Input: dimensioned drawing with shaded views. Units: mm. Origin: part minimum x, y, z. Coordinates: 2 decimals unless noted, no trailing zeros. Write each loop counter-clockwise with the first axis right and the second up, starting at its lowest first coordinate (ties: lowest second). Pieces come first, ordered by that corner, then holes. Notation, with made-up numbers: (77, -30) -> (136, -30) arc R22 ccw to (136, -16) -> close; hole circle Ø1 at (-24, 3). An arc over 180 degrees is marked (long way). One line per item, written item: value. Start each with the question number.
1. Section query B-B, the plane x = 123. Output: boundary loops of the cut face in (y, z), and give its area (3 significant figures).
2. Section query A-A, the plane y = 61. Output: boundary loops of the cut face in (x, z).
3. Section query C-C, the plane z = 914. Output: boundary loops of the cut face in (x, y) (1 decimal).
4. Section query D-D, the plane z = 535. Output: boundary loops of the cut face in (x, y).
5. First-contact query: P1, Ø1, axis at x = 142.5, z = 363.5, coming from the +Y side; P2, Ø2, axis at x = 125.5, z = 731.5, coming from the -Y side; P3, Ø2, axis at y = 54, z = 395, coming from the -X side; P4, Ø10, axis at x = 27.5, y = 89.5, coming from the -Z side. Flat tips, straight axial feed; report the tip coordinate or a pass-through.
6. Line query: line 1 (Y direction, x = 151, z = 382); line 2 (X direction, y = 35, z = 1002); line 3 (Y direction, x = 60, z = 213). Output: solid intervals per line, ascending.
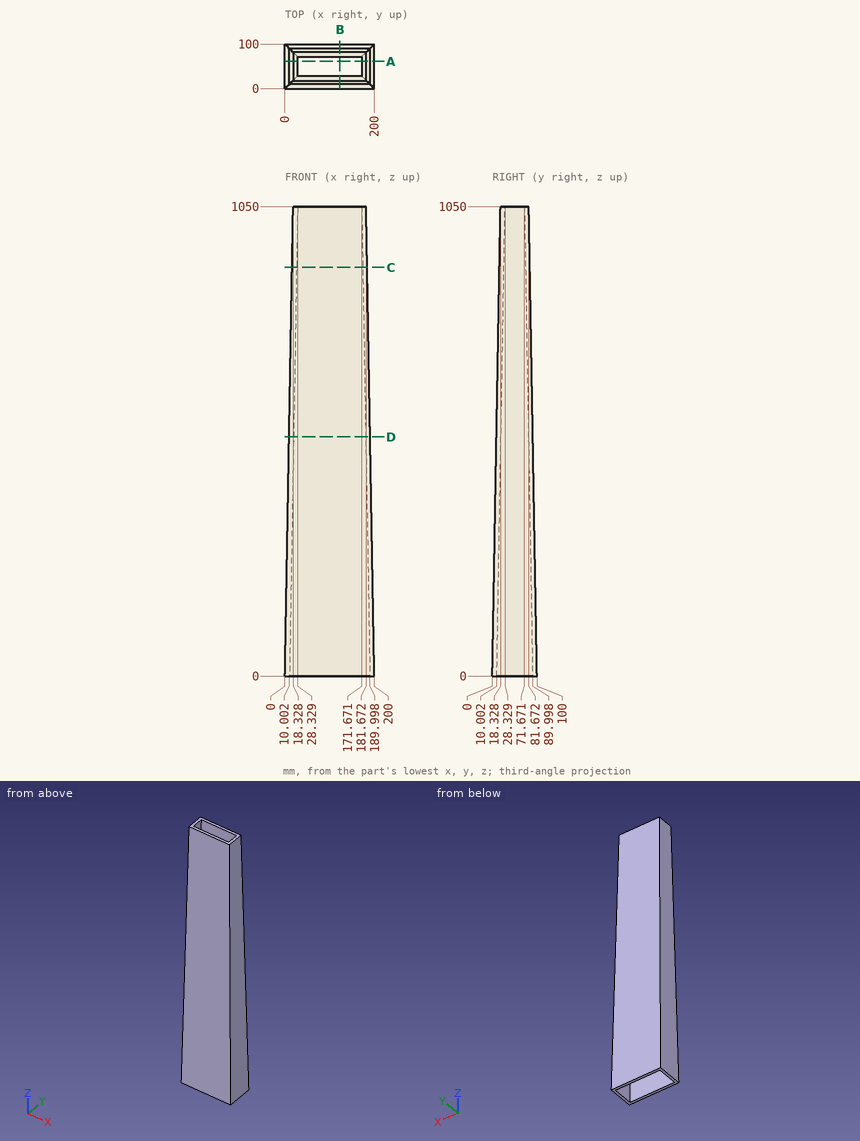
Computed values:
1. outline: (0, 0) -> (10, 0) -> (28.33, 1050) -> (18.33, 1050) -> close; (71.67, 1050) -> (90, 0) -> (100, 0) -> (81.67, 1050) -> close
1. area: 21,000 mm²
2. outline: (0, 0) -> (10, 0) -> (28.33, 1050) -> (18.33, 1050) -> close; (171.67, 1050) -> (190, 0) -> (200, 0) -> (181.67, 1050) -> close
3. outline: (16, 16) -> (184, 16) -> (184, 84) -> (16, 84) -> close; hole (26, 26) -> (174, 26) -> (174, 74) -> (26, 74) -> close
4. outline: (9.34, 9.34) -> (190.66, 9.34) -> (190.66, 90.66) -> (9.34, 90.66) -> close; hole (19.34, 19.34) -> (180.66, 19.34) -> (180.66, 80.66) -> (19.34, 80.66) -> close
5. P1: stops at y = 93.66
5. P2: stops at y = 12.75
5. P3: stops at x = 6.88
5. P4: stops at z = 0
6. line 1: y = 6.67 to 16.67, 83.33 to 93.33
6. line 2: x = 17.49 to 27.49, 172.51 to 182.51
6. line 3: y = 3.72 to 13.72, 86.28 to 96.28
